The model under review builds one solid part; all positions refer to its coordinate system, in mm. A direction names the side the tool comes from. Coordinates: 2 decimals unless noted, no trailing zeros. Answer in a Markdown table with one row per item.
from build123d import *

# Parameters (mm, degrees)
SKETCH5_R                = 6.05
CUT_EXTRUDE1_DEPTH       = 107.367288205
SKETCH7_R                = 1.65
CUT_EXTRUDE3_DEPTH       = 107.367288205
CUT_EXTRUDE4_DEPTH       = 107.367288205
FILLET1_R                = 6
CIRPATTERN1_COUNT        = 5
FILLET1_OF_CIRPATTERN1_R = 6


with BuildPart() as part:
    # Sketch3 → Revolve1 (revolve)
    with BuildSketch(Plane.XY, mode=Mode.PRIVATE) as revolve1_sk:
        Polygon((0, 0), (8, 0), (8, 66.5), (4.743746991, 66.5), (1.65, 75), (0, 75), align=None)
    revolve(revolve1_sk.sketch.rotate(Axis((0, 0, 0), (1, 0, 0)), 90), axis=Axis((0, 0, 0), (1, 0, 0)))

    # Sketch5 → Cut-Extrude1 (cut, through all)
    with BuildSketch(Plane(origin=(0, 0, 0), x_dir=(0, 0, -1), z_dir=(1, 0, 0))):
        Circle(SKETCH5_R)
    extrude(amount=CUT_EXTRUDE1_DEPTH, mode=Mode.SUBTRACT)

    # Sketch7 → Cut-Extrude3 (cut, through all)
    with BuildSketch(Plane(origin=(8, 0, 0), x_dir=(0, 0, -1), z_dir=(1, 0, 0))):
        with Locations((0, 60)):
            Circle(SKETCH7_R)
        with Locations((51.961524227, -30)):
            Circle(SKETCH7_R)
        with Locations((-51.961524227, -30)):
            Circle(SKETCH7_R)
        with Locations((10.825317547, 6.25)):
            Circle(SKETCH7_R)
        with Locations((0, -12.5)):
            Circle(SKETCH7_R)
        with Locations((-10.825317547, 6.25)):
            Circle(SKETCH7_R)
    extrude(amount=-CUT_EXTRUDE3_DEPTH, mode=Mode.SUBTRACT)

    # Sketch8 → Cut-Extrude4 (cut, through all)
    with BuildSketch(Plane(origin=(8, 0, 0), x_dir=(0, 0, -1), z_dir=(1, 0, 0))):
        with BuildLine():
            Line((2.264064275, 19.871437114), (5.99977033, 52.659308351))
            ThreePointArc((5.99977033, 52.659308351), (31.152618372, 42.877900702), (48.227947356, 21.978741861))
            Line((48.227947356, 21.978741861), (18.199225418, 8.293864853))
            ThreePointArc((18.199225418, 8.293864853), (11.755705046, 16.180339887), (2.264064275, 19.871437114))
        make_face()
    cut_extrude4 = extrude(amount=-CUT_EXTRUDE4_DEPTH, mode=Mode.SUBTRACT)

    # Fillet1
    fillet1_edges = [part.edges().sort_by_distance(p)[0] for p in [
        (4, 21.978741861, -48.227947356),
        (4, 8.293864853, -18.199225418),
        (4, 19.871437114, -2.264064275),
        (4, 52.659308351, -5.99977033),
    ]]
    fillet(fillet1_edges, radius=FILLET1_R)

    # CirPattern1: Cut-Extrude4 ×5 about axis
    cirpattern1_axis = Axis((0, 0, 0), (1, 0, 0))
    for i in range(1, CIRPATTERN1_COUNT):
        add(cut_extrude4.rotate(cirpattern1_axis, i * 360 / CIRPATTERN1_COUNT), mode=Mode.SUBTRACT)

    # Fillet1 of CirPattern1
    fillet1_of_cirpattern1_edges = [part.edges().sort_by_distance(p)[0] for p in [
        (4, 52.659308351, 5.99977033),
        (4, 19.871437114, 2.264064275),
        (4, 8.293864853, 18.199225418),
        (4, 21.978741861, 48.227947356),
        (4, 10.566500524, 51.936009345),
        (4, 3.987358688, 19.598494092),
        (4, -14.745546736, 13.511804152),
        (4, -39.075698851, 35.806281004),
        (4, -46.128851885, 26.098448685),
        (4, -17.407113919, 9.848471202),
        (4, -17.407113919, -9.848471202),
        (4, -46.128851885, -26.098448685),
        (4, -39.075698851, -35.806281004),
        (4, -14.745546736, -13.511804152),
        (4, 3.987358688, -19.598494092),
        (4, 10.566500524, -51.936009345),
    ]]
    fillet(fillet1_of_cirpattern1_edges, radius=FILLET1_OF_CIRPATTERN1_R)


solid = part.part
(1) To check wall thickness, follow line 1 (Y direction, x = 6.5, z = 0); line 2 (Y direction, x = 1, z = -25); line 3 (Y direction, x = 5.5, z = -2). State the ranges of each line that lie inside material, in increasing order. Write a range as [from, to].
Report:
| item | result |
|---|---|
| line 1 | [-66.5, -53], [-20, -14.15], [-10.85, -6.05], [6.05, 58.35], [61.65, 66.5] |
| line 2 | [-70.71, -27.28], [5.09, 11.39], [46.73, 70.71] |
| line 3 | [-66.47, -52.96], [-19.9, -5.71], [5.71, 66.47] |
(2) Insertion check: P1, Ø19.5, axis at y = 0, z = 0, coming from the -X side; P2, Ø1, axis at x = 5.5, z = -35, coming from the +Y side. Each pin has a flat end and moves straight along its axis. Give the tip position at first contact, or say it passes through.
Report:
| item | result |
|---|---|
| P1 | x = 0 |
| P2 | y = 56.85 |
(3) The part is to be moulded in two halves that separate along Y. For faces 1 (the cylindrical face through (3.944, -45.429, -23.423)), 2 (the cylindrical face through (4.06, 42.71, 31.38)), 3 (the cylindrical face through (0.813, 66.538, 34.608)), say which applies: +Y half, -Y half, draft (parallel to the pull), parting line (faces both ways), or undercut.
Report:
| item | result |
|---|---|
| face 1 | undercut |
| face 2 | undercut |
| face 3 | parting line |
(4) Take a section at A-A (z = 35). State how many separate pieces and enclosed holes the cut face has, then the cut area to 3 significant figures.
Report:
| item | result |
|---|---|
| separate pieces | 3 |
| enclosed holes | 0 |
| area | 430 mm^2 |
(5) Machinability: for faces 4 (the cylindrical face through (3.944, 2.991, 21.366)), 5 (the cylindrical face through (6.349, -56.073, 35.75)), which of the approach directions +Z, -Z, +X, -X, +Y, -Y give a long, thin tool a straight path to every point of the face, cutting with its end or side? Answer none if there is none.
Report:
| item | result |
|---|---|
| face 4 | +X, -X |
| face 5 | +X |
